Geometry check sheet. Reference: the model listing, model coordinates, mm. Round coordinates to 2 decimals unless told otherwise and drop trailing zeros. Write each loop counter-clockwise with the first axis right and the second up, starting at its lowest first coordinate (ties: lowest second). Pieces come first, ordered by that corner, then holes.
Autodesk Fusion 360 part; units mm, degrees
sketch "Skizze1" plane through (0, 0, 0) normal (0, 1, 0) x (1, 0, 0)
  line L0 (0, 0) -> (6, 0)
  line L1 (6, 0) -> (6, -6)
  line L2 (6, -6) -> (0, -6)
  line L3 (0, -6) -> (0, 0)
  dimension "d1" = 6
  dimension "d2" = 6
extrude "Extrusion1" add sketch "Skizze1" along normal blind 100
sketch "Skizze2" plane through (6, 0, 0) normal (1, 0, 0) x (0, 1, 0)
  line L0 (0, 6) -> (0, 0)
  line L1 (0, 0) -> (100, 0)
  line L2 (100, 0) -> (100, 6)
  line L3 (100, 6) -> (0, 6)
  point P0 (95, 3)
  point P1 (55, 3)
  dimension "d5" = 3
  dimension "d6" = 3
  dimension "d7" = 5
  dimension "d8" = 45
hole "Bohrung1" at (6, 95, 3) at (6, 55, 3) direction (-1, 0, 0) diameter 2.529 depth 30 tip angle 118
1. Section check A-A (y = 55). Record the cut outline in (x, z).
2. Depth check by flat-ended pin: pin 1 Ø2 at (y, z) = (95, 3) entering from -X; pin 2 Ø1.5 at (x, y) = (4, 39) entering from -Z. Enter the tip coordinate at first touch or a pass-through.
3. Section check B-B (z = 3). Record the cut outline in (x, y).
4. Scan lines: line 1 along Y through (x, z) = (5.4, 2.9); line 2 along Z through (x, y) = (3.95, 55); line 3 along Y through (x, z) = (2.5, 3.95). Record each from-to range of solid material in increasing order.
5. Section check C-C (x = 2.85). Record the cut outline in (y, z).
6. Release check for a two-part mould opening along Z. For faces 1 (the face through (2.958, 53.934, 2.32)), 2 (the face through (0, 49, 3)), 3 (the face through (3, 49, 6)) record: +Z half, -Z half, draft (parallel to the pull), parting line (faces both ways), or undercut.
Results below:
1. outline: (0, 0) - (6, 0) - (6, 1.74) - (0, 1.74) - close; (0, 4.26) - (6, 4.26) - (6, 6) - (0, 6) - close
2. pin 1: passes through
2. pin 2: stops at z = 0
3. outline: (0, 0) - (6, 0) - (6, 53.74) - (0, 53.74) - close; (0, 56.26) - (6, 56.26) - (6, 93.74) - (0, 93.74) - close; (0, 96.26) - (6, 96.26) - (6, 100) - (0, 100) - close
4. line 1: y = 0 to 53.74, 56.26 to 93.74, 96.26 to 100
4. line 2: z = 0 to 1.74, 4.26 to 6
4. line 3: y = 0 to 54.17, 55.83 to 94.17, 95.83 to 100
5. outline: (0, 0) - (100, 0) - (100, 6) - (0, 6) - close; hole circle Ø2.53 at (55, 3); hole circle Ø2.53 at (95, 3)
6. face 1: undercut
6. face 2: draft
6. face 3: +Z half
